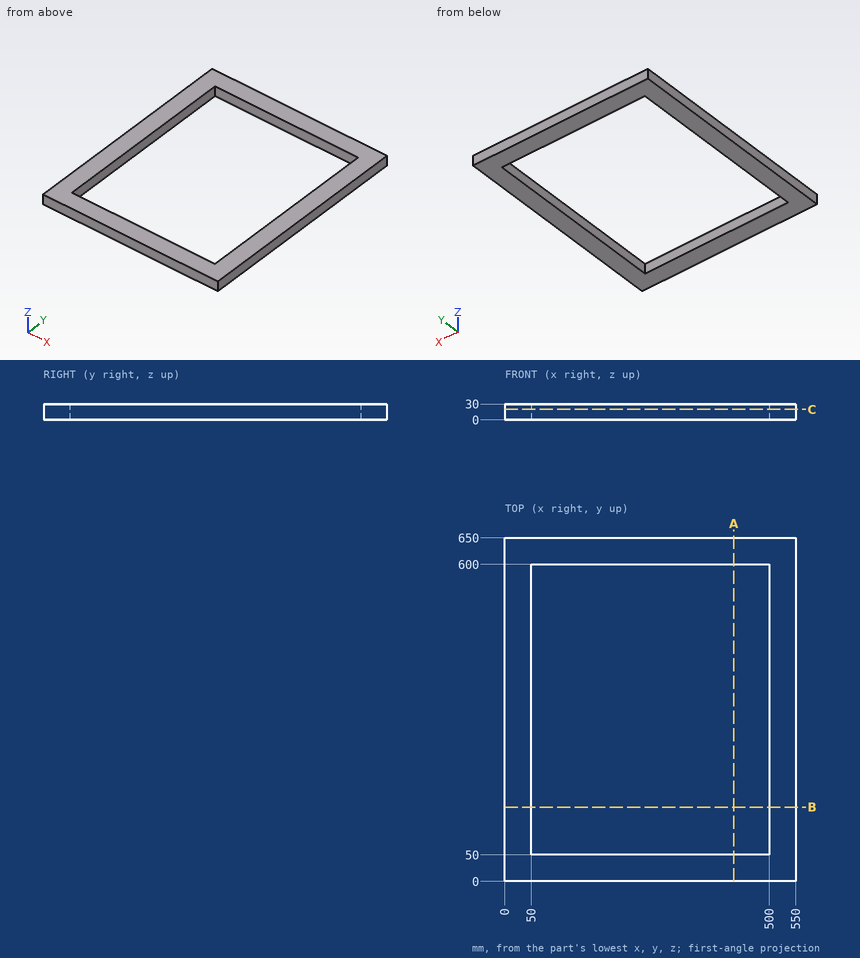
Drawing for the job (mm, zero at the part's lowest x, y, z). Round coordinates to 2 decimals unless told otherwise and drop trailing zeros. Loops run counter-clockwise (first coordinate to the right, second up) from the corner with the lowest first, then second, coordinate; pieces in that order, holes last. Notation, with made-up numbers: (86, 44.25) -> (96, 44.25) arc R26 ccw to (96, 80.25) -> close; hole circle Ø11 at (57.25, 47.5). An arc over 180 degrees is marked (long way). Answer as CSV lines item,"result". Start each with the question number.
1) Slice it at C-C (z = 20). List the corners of the cut face in (x, y), plus the area to 3 significant figures.
2) Slice it at B-B (y = 140.5). List the corners of the cut face in (x, z).
3) Slice it at A-A (x = 433.5). List the corners of the cut face in (y, z), plus the area to 3 significant figures.
4) Probe line 1 along X through (y, z) = (186, 13.5); line 2 along Y through (x, z) = (316.5, 28.5). List the from-to ranges inside material, lowest first.
Filled in:
1,outline,"(0, 0) -> (550, 0) -> (550, 650) -> (0, 650) -> close; hole (50, 50) -> (500, 50) -> (500, 600) -> (50, 600) -> close"
1,area,"110,000 mm2"
2,outline,"(0, 0) -> (50, 0) -> (50, 30) -> (0, 30) -> close; (500, 0) -> (550, 0) -> (550, 30) -> (500, 30) -> close"
3,outline,"(0, 0) -> (50, 0) -> (50, 30) -> (0, 30) -> close; (600, 0) -> (650, 0) -> (650, 30) -> (600, 30) -> close"
3,area,"3,000 mm2"
4,line 1,"x = 0 to 50, 500 to 550"
4,line 2,"y = 0 to 50, 600 to 650"
